Part model, mm, in its own coordinate system. A direction names the side the tool comes from. Coordinates: 2 decimals unless noted, no trailing zeros. Order: outer loops, then holes, each group sorted by start corner. A loop starts at its lowest first (then second) coordinate and runs counter-clockwise, first axis right, second up.
1) Pin check, flat tips, straight feed: pin 1 Ø1.1 at (x, y) = (68, 2) entering from -Z; pin 2 Ø1.5 at (x, y) = (108.5, 9.5) entering from -Z; pin 3 Ø3 at (x, y) = (55.5, 10) entering from -Z. Stop position of each tip, or through.
2) Cut at A-A (x = 63.5). List the corners of the cut face in (y, z) (3 decimals).
3) Tool access for faces 3 (the flat face through (90, 6, -171.45)), 4 (the flat face through (114.3, 10, -88)): list every direction of +Z, -Z, +X, -X, +Y, -Y with a clear straight run to the whole face (end or side of a thin tool).
4) Cut at B-B (z = -109). List the corners of the cut face in (x, y) (3 decimals).
5) Wall check: L1, parallel to X at y = 3, z = -6.35; L2, parallel to Z at x = 6.35, y = 9.5; L3, parallel to X at y = 5.5, z = -209.55. Give the ranges that are in metal, low to high.
6) Cut at C-C (x = 95.5). List the corners of the cut face in (y, z), and give its area (3 significant figures).
7) Mould opens along X. For faces 1 (the flat face through (6, 6, -215.9)), 2 (the flat face through (38, 8, -165.1)) say: +X half, -X half, draft (parallel to the pull), parting line (faces both ways), or undercut.
```python
from build123d import *

# Parameters (mm, degrees)
SKETCH2_W                   = 127
SKETCH2_H                   = 215.9
BOSS_EXTRUDE1_DEPTH         = 12.7
SKETCH5_W                   = 101.6
SKETCH5_H                   = 152.4
CUT_EXTRUDE3_DEPTH          = 5.588
SKETCH6_W                   = 101.6
SKETCH6_H                   = 44.45
CUT_EXTRUDE4_DEPTH          = 251.804904258
SKETCH8_R                   = 8.980256121
CUT_EXTRUDE6_DEPTH          = 251.804904258
SKETCH9_W                   = 95.25
SKETCH9_H                   = 146.05
CUT_EXTRUDE7_DEPTH          = 3.302
CUT_EXTRUDE8_DEPTH          = 3.81
F_32_0_116_DIAMETER_HOLE1_D = 2.9464
SKETCH18_R                  = 3.175
CUT_EXTRUDE9_DEPTH          = 5.588
FILLET5_R                   = 6.35
FILLET7_R                   = 6.35
FILLET8_R                   = 6.35
FILLET10_R                  = 6.35
FILLET11_R                  = 6.35


with BuildPart() as part:
    # Sketch2 → Boss-Extrude1 (new body)
    with BuildSketch(Plane(origin=(0, 0, 0), x_dir=(1, 0, 0), z_dir=(0, 1, 0))):
        with Locations((63.5, 107.95)):
            Rectangle(SKETCH2_W, SKETCH2_H)
    extrude(amount=BOSS_EXTRUDE1_DEPTH)

    # Sketch5 → Cut-Extrude3 (cut)
    with BuildSketch(Plane(origin=(0, 12.7, 0), x_dir=(1, 0, 0), z_dir=(0, 1, 0))):
        with Locations((63.5, 88.9)):
            Rectangle(SKETCH5_W, SKETCH5_H)
    extrude(amount=-CUT_EXTRUDE3_DEPTH, mode=Mode.SUBTRACT)

    # Sketch6 → Cut-Extrude4 (cut, through all)
    with BuildSketch(Plane(origin=(0, 12.7, 0), x_dir=(1, 0, 0), z_dir=(0, 1, 0))):
        with Locations((63.5, 193.675)):
            Rectangle(SKETCH6_W, SKETCH6_H)
    extrude(amount=-CUT_EXTRUDE4_DEPTH, mode=Mode.SUBTRACT)

    # Sketch8 → Cut-Extrude6 (cut, through all)
    with BuildSketch(Plane(origin=(0, 12.7, 0), x_dir=(1, 0, 0), z_dir=(0, 1, 0))):
        with Locations((63.5, 171.45)):
            Circle(SKETCH8_R)
    extrude(amount=-CUT_EXTRUDE6_DEPTH, mode=Mode.SUBTRACT)

    # Sketch9 → Cut-Extrude7 (cut)
    with BuildSketch(Plane(origin=(0, 7.112, 0), x_dir=(1, 0, 0), z_dir=(0, 1, 0))):
        with Locations((63.5, 92.075)):
            Rectangle(SKETCH9_W, SKETCH9_H)
    extrude(amount=-CUT_EXTRUDE7_DEPTH, mode=Mode.SUBTRACT)

    # Sketch11 → Cut-Extrude8 (cut)
    with BuildSketch(Plane(origin=(0, 3.81, 0), x_dir=(1, 0, 0), z_dir=(0, 1, 0))):
        with BuildLine():
            Line((74.93, 155.575), (52.07, 155.575))
            ThreePointArc((52.07, 155.575), (50.165, 157.48), (52.07, 159.385))
            Line((52.07, 159.385), (74.93, 159.385))
            ThreePointArc((74.93, 159.385), (76.835, 157.48), (74.93, 155.575))
        make_face()
    extrude(amount=-CUT_EXTRUDE8_DEPTH, mode=Mode.SUBTRACT)

    # #32 (0.116) Diameter Hole1 (through all)
    with Locations(Plane(origin=(0, 12.7, 0), x_dir=(1, 0, 0), z_dir=(0, 1, 0))):
        with Locations((6.35, 209.55), (120.65, 209.55), (120.65, 6.35), (6.35, 6.35), (6.35, 146.05), (120.65, 146.05)):
            Hole(F_32_0_116_DIAMETER_HOLE1_D / 2)

    # Sketch18 → Cut-Extrude9 (cut)
    with BuildSketch(Plane(origin=(0, 12.7, 0), x_dir=(1, 0, 0), z_dir=(0, 1, 0))):
        with Locations((12.7, 165.1)):
            Circle(SKETCH18_R)
        with Locations((114.3, 165.1)):
            Circle(SKETCH18_R)
        with Locations((114.3, 12.7)):
            Circle(SKETCH18_R)
        with Locations((12.7, 12.7)):
            Circle(SKETCH18_R)
    extrude(amount=-CUT_EXTRUDE9_DEPTH, mode=Mode.SUBTRACT)

    # Fillet5
    fillet5_edges = [part.edges().sort_by_distance(p)[0] for p in [
        (12.7, 9.906, -15.875),
        (15.875, 9.906, -12.7),
        (114.3, 9.906, -15.875),
        (111.125, 9.906, -12.7),
        (111.125, 9.906, -165.1),
        (114.3, 9.906, -161.925),
        (15.875, 9.906, -165.1),
        (12.7, 9.906, -161.925),
    ]]
    fillet(fillet5_edges, radius=FILLET5_R)

    # Fillet7
    fillet7_edges = [part.edges().sort_by_distance(p)[0] for p in [
        (12.7, 6.35, -171.45),
        (114.3, 6.35, -171.45),
    ]]
    fillet(fillet7_edges, radius=FILLET7_R)

    # Fillet8
    fillet8_edges = [part.edges().sort_by_distance(p)[0] for p in [
        (15.875, 5.461, -19.05),
        (111.125, 5.461, -19.05),
    ]]
    fillet(fillet8_edges, radius=FILLET8_R)

    # Fillet10
    # the kernel refuses this fillet: 6.35 mm, written as the material it adds along each edge
    with BuildSketch(Plane(origin=(111.125, 7.112, -165.1), x_dir=(-1, 0, 0), z_dir=(0, -1, 0))) as fillet10_piece_1:
        with BuildLine():
            CenterArc((FILLET10_R, -FILLET10_R), FILLET10_R, 90, 90)
            Line((0, -FILLET10_R), (0, 0))
            Line((0, 0), (FILLET10_R, 0))
        make_face()
    extrude(amount=3.302)

    # Fillet11
    # the kernel refuses this fillet: 6.35 mm, written as the material it adds along each edge
    with BuildSketch(Plane(origin=(15.875, 7.112, -165.1), x_dir=(1, 0, 0), z_dir=(0, -1, 0))) as fillet11_piece_1:
        with BuildLine():
            CenterArc((FILLET11_R, FILLET11_R), FILLET11_R, 180, 90)
            Line((0, FILLET11_R), (0, 0))
            Line((0, 0), (FILLET11_R, 0))
        make_face()
    extrude(amount=3.302)


solid = part.part
```
Geometry check:
1. pin 1: stops at z = -164.02
1. pin 2: stops at z = -171.58
1. pin 3: stops at z = -171.45
2. outline: (0, -162.47) - (3.81, -162.47) - (3.81, -159.385) - (0, -159.385) - close; (0, -155.575) - (3.81, -155.575) - (3.81, -19.05) - (7.112, -19.05) - (7.112, -12.7) - (12.7, -12.7) - (12.7, 0) - (0, 0) - close
3. face 3: -Z, +Y, -Y
3. face 4: +Y
4. outline: (0, 0) - (127, 0) - (127, 12.7) - (114.3, 12.7) - (114.3, 7.112) - (111.125, 7.112) - (111.125, 3.81) - (15.875, 3.81) - (15.875, 7.112) - (12.7, 7.112) - (12.7, 12.7) - (0, 12.7) - close
5. L1: x = 0 to 4.88, 7.82 to 119.18, 122.12 to 127
5. L2: z = -215.9 to -211.02, -208.08 to -147.52, -144.58 to -7.82, -4.88 to 0
5. L3: x = 0 to 4.88, 7.82 to 12.7, 114.3 to 119.18, 122.12 to 127
6. outline: (0, -171.45) - (12.7, -171.45) - (12.7, -165.1) - (3.81, -165.1) - (3.81, -19.05) - (7.11, -19.05) - (7.11, -12.7) - (12.7, -12.7) - (12.7, 0) - (0, 0) - close
6. area: 844 mm2
7. face 1: draft
7. face 2: undercut
